Can you work these out from the model? Positions are in its coordinate system, mm. A direction names the side the tool comes from. Coordinates: 2 decimals unless noted, no trailing zeros. Loops run counter-clockwise (first coordinate to the right, second up) from the corner with the lowest first, then second, coordinate; pieces in that order, holes last. Notation, with made-up numbers: M 84.5,80 L 95.5,80 A5 ccw 95.5,84 Z; hole C 37.25,52.5 d11. An arc over 180 degrees is marked long. Answer as a JSON object with one key per item and string values. Group by question number.
Item 1: Suppose I cut it at A-A (z = -14). Write out the boundary of the cut face in (x, y).
Item 2: We'd pull the mould along X, two halves only. Please class faces 5 (the flat face through (25, -8.4, -14.4)), 6 (the flat face through (108, -12.45, 0)), 7 (the flat face through (47.5, 5, -16)): +X half, -X half, draft (parallel to the pull), parting line (faces both ways), or undercut.
Item 3: Suppose I cut it at B-B (x = 70.5). Write out the boundary of the cut face in (y, z), then the cut area to 3 significant figures.
Item 4: Which directions (+Z, -Z, +X, -X, +Y, -Y) give clear straight access to the entire face, cutting with the end or side of a thin tool? Please do faces 1 (the flat face through (25, 8, -14.4)), 2 (the cylindrical face through (12.422, 3.584, -2.285)), 3 (the cylindrical face through (110.297, 11.309, -11.247)), 4 (the flat face through (25, 8.5, 14.4)).
Item 5: If I drill on line 1 (Y direction, x = 11.5, z = 0); line 2 (X direction, y = -7, z = 3.5); line 3 (Y direction, x = 62, z = 2), over which ranges is the centre line in solid material (lowest first)?
Item 6: I'm going to push flat-ended pins straight in: pin 1 Ø4 at (y, z) = (1.5, 13.5) entering from +X; pin 2 Ø6 at (x, z) = (32.5, 1.5) entering from +Y; pin 3 Ø1.6 at (y, z) = (17, -2) entering from -X; pin 4 Ø12 at (y, z) = (2.5, -4) entering from +X. Where does each tip first touch, or does it pass through?
```python
from build123d import *

# Parameters (mm, degrees)
SKETCH1_W                  = 125
SKETCH1_H                  = 17.5
SKETCH3_R                  = 15.75
CUT_EXTRUDE1_DEPTH         = 4
CUT_EXTRUDE2_DEPTH         = 25
CUT_EXTRUDE2_DEPTH_BACK    = 25
SKETCH5_OUTSIDE_W          = 63.888
SKETCH5_OUTSIDE_H          = 63.888
CUT_EXTRUDE3_DEPTH         = 25
SKETCH6_W                  = 1.6
SKETCH6_H                  = 12.966966859
M10X1_5_TAPPED_HOLE1_D     = 8.5
M10X1_5_TAPPED_HOLE1_DEPTH = 24.5
M10X1_5_TAPPED_HOLE1_TIP   = 2.553657631


with BuildPart() as part:
    # Sketch1 → Revolve1 (revolve)
    with BuildSketch(Plane.XY, mode=Mode.PRIVATE) as revolve1_sk:
        with Locations((62.5, 8.75)):
            Rectangle(SKETCH1_W, SKETCH1_H)
    revolve(revolve1_sk.sketch.rotate(Axis((0, 0, 0), (-1, 0, 0)), 90), axis=Axis((0, 0, 0), (-1, 0, 0)))

    # Sketch3 → Cut-Extrude1 (cut)
    with BuildSketch(Plane(origin=(125, 0, 0), x_dir=(0, 0, -1), z_dir=(1, 0, 0))):
        Circle(SKETCH3_R)
    extrude(amount=-CUT_EXTRUDE1_DEPTH, mode=Mode.SUBTRACT)

    # Sketch4 → Cut-Extrude2 (cut, two sides: drawn at the far end of the back side and taken through both)
    with BuildSketch(Plane(origin=(121, 0, 0), x_dir=(0, 0, -1), z_dir=(1, 0, 0)).offset(-CUT_EXTRUDE2_DEPTH_BACK)):
        with BuildLine():
            Line((-8.45, 12.45), (8.45, 12.45))
            ThreePointArc((8.45, 12.45), (11.278427125, 11.278427125), (12.45, 8.45))
            Line((12.45, 8.45), (12.45, -8.45))
            ThreePointArc((12.45, -8.45), (11.278427125, -11.278427125), (8.45, -12.45))
            Line((8.45, -12.45), (-8.45, -12.45))
            ThreePointArc((-8.45, -12.45), (-11.278427125, -11.278427125), (-12.45, -8.45))
            Line((-12.45, -8.45), (-12.45, 8.45))
            ThreePointArc((-12.45, 8.45), (-11.278427125, 11.278427125), (-8.45, 12.45))
        make_face()
    extrude(amount=CUT_EXTRUDE2_DEPTH + CUT_EXTRUDE2_DEPTH_BACK, mode=Mode.SUBTRACT)

    # Sketch5 outside → Cut-Extrude3 (cut)
    with BuildSketch(Plane.ZY):
        Rectangle(SKETCH5_OUTSIDE_W, SKETCH5_OUTSIDE_H)
        Polygon((9.237604307, 16), (-9.237604307, 16), (-18.475208614, 0), (-9.237604307, -16), (9.237604307, -16), (18.475208614, 0), align=None, mode=Mode.SUBTRACT)
    extrude(amount=-CUT_EXTRUDE3_DEPTH, mode=Mode.SUBTRACT)

    # Sketch6 → Cut-Revolve1 (revolve, cut)
    with BuildSketch(Plane(origin=(0, 0, 0), x_dir=(1, 0, 0), z_dir=(0, 1, 0))):
        with Locations((48.3, 22.98348343)):
            Rectangle(SKETCH6_W, SKETCH6_H)
    revolve(axis=Axis((0, 0, 0), (1, 0, 0)), mode=Mode.SUBTRACT)

    # M10x1.5 Tapped Hole1
    with Locations(Plane.ZY):
        with Locations((0, 0)):
            Hole(M10X1_5_TAPPED_HOLE1_D / 2, depth=M10X1_5_TAPPED_HOLE1_DEPTH)
            with Locations((0, 0, -(M10X1_5_TAPPED_HOLE1_DEPTH + M10X1_5_TAPPED_HOLE1_TIP / 2))):  # 118° drill point
                Cone(0, M10X1_5_TAPPED_HOLE1_D / 2, M10X1_5_TAPPED_HOLE1_TIP, mode=Mode.SUBTRACT)


solid = part.part
```
From the geometry:
{
 "1": {"outline": "M 0,-7.75 L 25,-7.75 L 25,-10.5 L 47.5,-10.5 L 47.5,-8.73 L 49.1,-8.73 L 49.1,-10.5 L 125,-10.5 L 125,-7.22 L 121,-7.22 L 121,7.22 L 125,7.22 L 125,10.5 L 49.1,10.5 L 49.1,8.73 L 47.5,8.73 L 47.5,10.5 L 25,10.5 L 25,7.75 L 0,7.75 Z"},
 "2": {"face 5": "-X half", "face 6": "draft", "face 7": "undercut"},
 "3": {"outline": "C 0,0 d35", "area": "962 mm2"},
 "4": {"face 1": "-Z, -X, +Y", "face 2": "-X", "face 3": "+X", "face 4": "+Z, -X, +Y"},
 "5": {"line 1": "-16 to -4.25, 4.25 to 16", "line 2": "0 to 96", "line 3": "-17.39 to 17.39"},
 "6": {"pin 1": "x = 121", "pin 2": "y = 17.5", "pin 3": "x = 25", "pin 4": "x = 96"}
}
